Verification items for the finished model (mm, model axes). Coordinates: 2 decimals unless noted, no trailing zeros. Loops run counter-clockwise (first coordinate to the right, second up) from the corner with the lowest first, then second, coordinate; pieces in that order, holes last. Notation, with made-up numbers: (20.25, -33.5) -> (28.25, -33.5) arc R31 ccw to (28.25, -5.5) -> close; hole circle Ø3 at (-19.5, -21). An arc over 180 degrees is marked (long way). Answer as a JSON object with one key per item and string values. Group by question number.
Q1. Cross-section at A-A on z = 9. Record the boundary of the cut face in (x, y), and give its area (3 significant figures).
Q2. Cross-section at C-C on y = -0.7. Record the boundary of the cut face in (x, z), and give its area (3 significant figures).
Q3. Cross-section at B-B on x = 23. Record the boundary of the cut face in (y, z).
Q4. Scan lines: L1, parallel to Y at x = 18, z = 9; L2, parallel to Y at x = 23, z = 3.25. Record each from-to range of solid material in increasing order.
Q5. Gauge pin test, flat end, axial feed: pin 1 Ø1 at (x, z) = (23.5, 4.5) entering from +Y. Record the tip position at first contact, or that the pin passes through.
```python
from build123d import *

# Parameters (mm, degrees)
F0_W        = 30.988
F0_H        = 11.2268
F1_DEPTH    = 1.857375
F3_T1_DEPTH = 119.4307056724
F2_W        = 30.988
F2_H        = 11.2268
F4_DEPTH    = 2.794


# Not quite as in the source:
# - a fillet or chamfer that OpenCascade refuses, or shapes differently, is made with other operations: its cross-section is extruded or revolved along the edge and cut away or added


with BuildPart() as f1:
    # F0 (on Front) → F1 (new body)
    with BuildSketch(Plane.XZ):
        with Locations((15.494, 5.6134)):
            Rectangle(F0_W, F0_H)
    extrude(amount=F1_DEPTH)

    # F3: fillet of radius 127 on 1 edges, made by hand

    # F3_s2 → F3_t1 (cut)
    with BuildSketch(Plane.XY.offset(-54.1019528362)):
        with BuildLine():
            ThreePointArc((30.988, -1.857375), (20.2073897896, -0.4651957464), (9.3472188655, 0))
            Line((9.3472188655, 0), (30.988, 0))
            Line((30.988, 0), (30.988, -1.857375))
        make_face()
    extrude(amount=F3_T1_DEPTH, mode=Mode.SUBTRACT)

    # F2 (on face) → F4 (join)
    with BuildSketch(Plane.XZ.offset(1.857375)):
        with Locations((15.494, 5.6134)):
            Rectangle(F2_W, F2_H)
    extrude(amount=F4_DEPTH)


solid = f1.part
```
Computed values:
{
 "1": {"outline": "(0, -4.65) -> (30.99, -4.65) -> (30.99, -1.86) arc R127 ccw to (9.35, 0) -> (0, 0) -> close", "area": "131 mm²"},
 "2": {"outline": "(0, 0) -> (22.66, 0) -> (22.66, 11.23) -> (0, 11.23) -> close", "area": "254 mm²"},
 "3": {"outline": "(-4.65, 0) -> (-0.74, 0) -> (-0.74, 11.23) -> (-4.65, 11.23) -> close"},
 "4": {"L1": "y = -4.65 to -0.3", "L2": "y = -4.65 to -0.74"},
 "5": {"pin 1": "stops at y = -0.74"}
}
